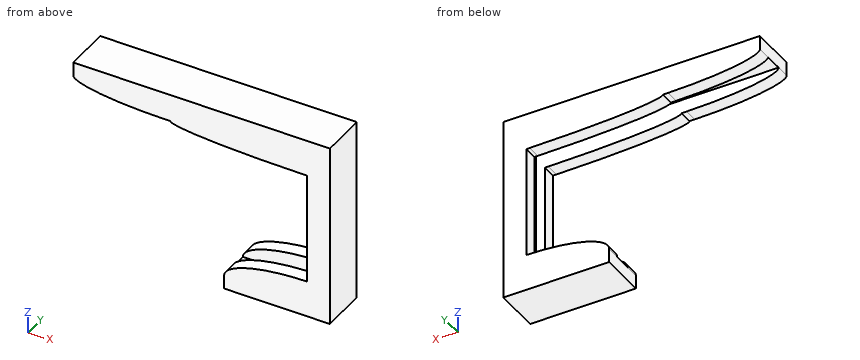
```python
from build123d import *

# Parameters (mm, degrees)
SKETCH1_W           = 27.9
SKETCH1_H           = 20.2
BOSS_EXTRUDE2_DEPTH = 5
CUT_EXTRUDE3_DEPTH  = 5
SKETCH5_W           = 17.2
SKETCH5_H           = 2
CUT_EXTRUDE4_DEPTH  = 26.4
FILLET1_SIZE        = 2.5
FILLET1_SIZE_2      = 9
FILLET2_SIZE        = 9
FILLET2_SIZE_2      = 2.5
FILLET3_SIZE        = 1
FILLET3_SIZE_2      = 14.5
FILLET4_DEPTH       = 1.5
FILLET5_START       = 3.5
FILLET5_DEPTH       = 1.5
FILLET6_DEPTH       = 1.5


with BuildPart() as part:
    # Sketch1 → Boss-Extrude2 (new body)
    with BuildSketch(Plane(origin=(0, 0, 0), x_dir=(1, 0, 0), z_dir=(0, 1, 0))):
        with Locations((-55.325764497, -25.209039536)):
            Rectangle(SKETCH1_W, SKETCH1_H)
    extrude(amount=BOSS_EXTRUDE2_DEPTH)

    # Sketch4 → Cut-Extrude3 (cut)
    with BuildSketch(Plane(origin=(0, 5, 0), x_dir=(1, 0, 0), z_dir=(0, 1, 0))):
        Polygon((-69.275764497, -32.309039536), (-58.719837606, -32.309039536), (-58.719837606, -31.309039536), (-43.875764497, -31.309039536), (-43.875764497, -19.109039536), (-52.875764497, -19.109039536), (-52.875764497, -15.109039536), (-69.275764497, -15.109039536), align=None)
    extrude(amount=-CUT_EXTRUDE3_DEPTH, mode=Mode.SUBTRACT)

    # Sketch5 → Cut-Extrude4 (cut)
    with BuildSketch(Plane.ZY.offset(69.275764497)):
        with Locations((25.209039536, 2.5)):
            Rectangle(SKETCH5_W, SKETCH5_H)
    extrude(amount=-CUT_EXTRUDE4_DEPTH, mode=Mode.SUBTRACT)

    # Fillet1
    # a fillet whose section is not a circle: 9, 2.5 mm, written as the material it takes off along each edge
    with BuildSketch(Plane(origin=(-52.875764497, 27.5, 19.109039536), x_dir=(0, 0, -1), z_dir=(0, -1, 0))) as fillet1_piece_1_section:
        with BuildLine():
            Bezier((FILLET1_SIZE, 0), (0, 0), (0, FILLET1_SIZE_2), weights=[1, 0.707106781, 1])
            Line((0, FILLET1_SIZE_2), (0, 0))
            Line((0, 0), (FILLET1_SIZE, 0))
        make_face()
    fillet1_piece_1 = extrude(amount=46.5, mode=Mode.PRIVATE)
    fillet1_piece_1 = split(fillet1_piece_1, bisect_by=Plane(origin=(-52.875764497, 1.5, 19.109039536), z_dir=(0, 1, 0)), keep=Keep.TOP, mode=Mode.PRIVATE)
    add(fillet1_piece_1, mode=Mode.SUBTRACT)

    # Fillet2
    # a fillet whose section is not a circle: 9, 2.5 mm, written as the material it takes off along each edge
    with BuildSketch(Plane(origin=(-52.875764497, 24, 19.109039536), x_dir=(1, 0, 0), z_dir=(0, -1, 0))) as fillet2_piece_1:
        with BuildLine():
            Bezier((FILLET2_SIZE, 0), (0, 0), (0, -FILLET2_SIZE_2), weights=[1, 0.707106781, 1])
            Line((0, -FILLET2_SIZE_2), (0, 0))
            Line((0, 0), (FILLET2_SIZE, 0))
        make_face()
    extrude(amount=46.5, mode=Mode.SUBTRACT)

    # Fillet3
    # a fillet whose section is not a circle: 14.5, 1 mm, written as the material it takes off along each edge
    with BuildSketch(Plane(origin=(-58.719837606, 41.25, 31.309039536), x_dir=(0, 0, 1), z_dir=(0, -1, 0))) as fillet3_piece_1_section:
        with BuildLine():
            Bezier((FILLET3_SIZE, 0), (0, 0), (0, -FILLET3_SIZE_2), weights=[1, 0.707106781, 1])
            Line((0, -FILLET3_SIZE_2), (0, 0))
            Line((0, 0), (FILLET3_SIZE, 0))
        make_face()
    fillet3_piece_1 = extrude(amount=74, mode=Mode.PRIVATE)
    fillet3_piece_1 = split(fillet3_piece_1, bisect_by=Plane(origin=(-58.719837606, 1.5, 31.309039536), z_dir=(0, 1, 0)), keep=Keep.TOP, mode=Mode.PRIVATE)
    add(fillet3_piece_1, mode=Mode.SUBTRACT)

    # Fillet4: read off the stored shape, not the designer's step
    # Fillet4 outline → Fillet4 (cut)
    with BuildSketch(Plane(origin=(0, 0, 0), x_dir=(1, 0, 0), z_dir=(0, 1, 0))):
        with BuildLine():
            add(Edge.make_bspline(
                [(-44.219837606, -31.309039536), (-58.719837606, -31.309039536), (-58.719837606, -32.309039536)],
                knots=[0, 0, 0, 1, 1, 1], degree=2, weights=[1, 0.707106781, 1]))
            Line((-44.219837606, -31.309039536), (-58.719837606, -31.309039536))
            Line((-58.719837606, -31.309039536), (-58.719837606, -32.309039536))
        make_face()
    extrude(amount=FILLET4_DEPTH, mode=Mode.SUBTRACT)

    # Fillet5: read off the stored shape, not the designer's step
    # Fillet5 outline → Fillet5 (cut)
    with BuildSketch(Plane(origin=(0, 0, 0), x_dir=(1, 0, 0), z_dir=(0, 1, 0)).offset(FILLET5_START)):
        with BuildLine():
            add(Edge.make_bspline(
                [(-59.275764497, -32.309039536), (-69.275764497, -32.309039536), (-69.275764497, -33.809039536)],
                knots=[0, 0, 0, 1, 1, 1], degree=2, weights=[1, 0.707106781, 1]))
            Line((-59.275764497, -32.309039536), (-69.275764497, -32.309039536))
            Line((-69.275764497, -32.309039536), (-69.275764497, -33.809039536))
        make_face()
    extrude(amount=FILLET5_DEPTH, mode=Mode.SUBTRACT)

    # Fillet6: read off the stored shape, not the designer's step
    # Fillet6 outline → Fillet6 (cut)
    with BuildSketch(Plane(origin=(0, 0, 0), x_dir=(1, 0, 0), z_dir=(0, 1, 0))):
        with BuildLine():
            add(Edge.make_bspline(
                [(-59.275764497, -32.309039536), (-69.275764497, -32.309039536), (-69.275764497, -33.809039536)],
                knots=[0, 0, 0, 1, 1, 1], degree=2, weights=[1, 0.707106781, 1]))
            Line((-59.275764497, -32.309039536), (-69.275764497, -32.309039536))
            Line((-69.275764497, -32.309039536), (-69.275764497, -33.809039536))
        make_face()
    extrude(amount=FILLET6_DEPTH, mode=Mode.SUBTRACT)


solid = part.part
```
Geometry: final body of the model. Coordinates: model frame, mm. Round coordinates to 2 decimals unless told otherwise and drop trailing zeros. Order: outer loops, then holes, each group sorted by start corner. A loop starts at its lowest first (then second) coordinate and runs counter-clockwise, first axis right, second up. Notation, with made-up numbers: M 7.5,37.5 L 33.5,37.5 A35 cw 33.5,73.5 Z; hole C -22.75,-2.5 d3. An arc over 180 degrees is marked long. Use one line per item in the form item = value. Start each with the question number.
Q1. Cut plane B-B (y = 2.45). Return loops of the section in (x, z).
Q2. Pin query (flat end, axial travel): pin 1 Ø1.6 at (y, z) = (1, 25.5) entering from -X; pin 2 Ø1 at (y, z) = (2.5, 28) entering from -X; pin 3 Ø0.5 at (y, z) = (3, 15.5) entering from -X. Return the tip coordinate at first contact, or that it passes through.
Q3. Material intervals for line 1 (Z direction, x = -47, y = 2.95); line 2 (Y direction, x = -43.75, z = 33.75); line 3 (Z direction, x = -63.75, y = 3.3), sorted ascending. Write a range as [from, to].
Q4. Cut plane A-A (z = 30.75). Return loops of the section in (x, y), and give its area (3 significant figures).
Geometry results:
q1.outline = M -69.28,33.81 L -42.88,33.81 L -42.88,16.61 L -52.88,16.61 L -52.88,15.11 L -41.38,15.11 L -41.38,35.31 L -69.28,35.31 Z
q2.pin_1 = -43.88
q2.pin_2 = -42.88
q2.pin_3 = -52.88
q3.line_1 = [15.11, 16.61], [33.81, 35.31]
q3.line_2 = [0, 1.5], [3.5, 5]
q3.line_3 = [33.81, 35.31]
q4.outline = M -43.88,0 L -41.38,0 L -41.38,5 L -43.88,5 L -43.88,3.5 L -42.88,3.5 L -42.88,1.5 L -43.88,1.5 Z
q4.area = 10.5 mm^2
